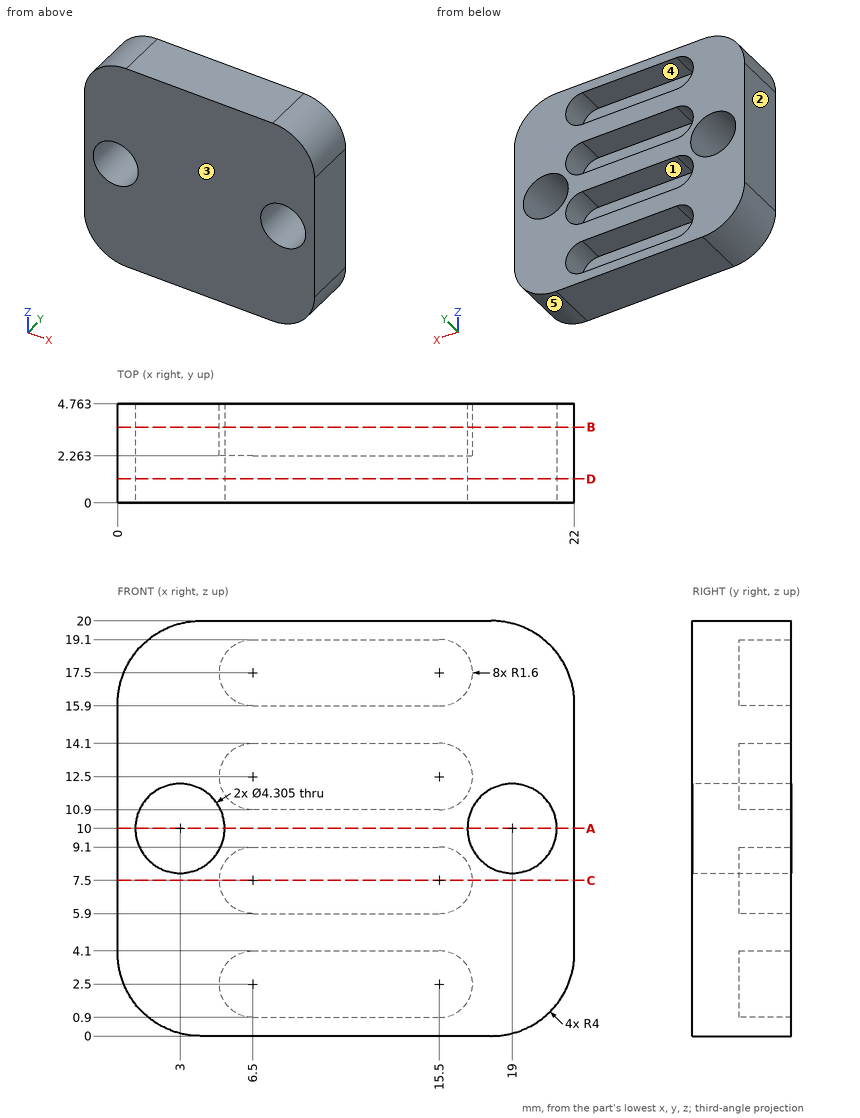
Print and shaded views of the part. All mm, measured from the part's lowest x, y and z. A direction names the side the tool comes from. Give positions to 0.01 mm unless a question says otherwise; leave off trailing zeros. Loops run counter-clockwise (first coordinate to the right, second up) from the corner with the lowest first, then second, coordinate; pieces in that order, holes last. Notation, with made-up numbers: (13.5, 8) -> (40.5, 8) arc R28 ccw to (40.5, 31) -> close; hole circle Ø4 at (-3, -35.75). An arc over 180 degrees is marked (long way). Use a Markdown table: item, result.
1. Which spindle directions (+Z, -Z, +X, -X, +Y, -Y) get a long thin tool onto all of the face, cutting with end or side? Do the marked faces 4 and 5. Say none if no direction does.
Check result:
| item | result |
|---|---|
| face 4 | +Y |
| face 5 | -Z, +X, +Y, -Y |
2. Mould opens along X. For the marked faces 1, 2 and 3 say: pulls with the +X half, pulls with the -X half, needs draft (parallel to the pull), parting line crosses it, or undercut.
Check result:
| item | result |
|---|---|
| face 1 | undercut |
| face 2 | pulls with the -X half |
| face 3 | needs draft |
3. Wall check: L1, parallel to X at y = 1.15, z = 10; L2, parallel to Z at x = 7.25, y = 2.7; L3, parallel to Y at x = 8.5, z = 18.5. Give the ranges that are in metal, low to high. Write a range as [from, to].
Check result:
| item | result |
|---|---|
| L1 | x = [0, 0.85], [5.15, 16.85], [21.15, 22] |
| L2 | z = [0, 0.9], [4.1, 5.9], [9.1, 10.9], [14.1, 15.9], [19.1, 20] |
| L3 | y = [0, 2.26] |
4. Slice it at C-C (z = 7.5). List the corners of the cut face in (x, y).
Check result:
| item | result |
|---|---|
| outline | (0, 0) -> (22, 0) -> (22, 4.76) -> (17.1, 4.76) -> (17.1, 2.26) -> (4.9, 2.26) -> (4.9, 4.76) -> (0, 4.76) -> close |
5. Slice it at A-A (z = 10). List the corners of the cut face in (x, y).
Check result:
| item | result |
|---|---|
| outline | (0, 0) -> (0.85, 0) -> (0.85, 4.76) -> (0, 4.76) -> close; (5.15, 0) -> (16.85, 0) -> (16.85, 4.76) -> (5.15, 4.76) -> close; (21.15, 0) -> (22, 0) -> (22, 4.76) -> (21.15, 4.76) -> close |
6. Slice it at D-D (y = 1.15). List the corners of the cut face in (x, z) (1 decimal).
Check result:
| item | result |
|---|---|
| outline | (0, 4) arc R4 ccw to (4, 0) -> (18, 0) arc R4 ccw to (22, 4) -> (22, 16) arc R4 ccw to (18, 20) -> (4, 20) arc R4 ccw to (0, 16) -> close; hole circle Ø4.3 at (3, 10); hole circle Ø4.3 at (19, 10) |
7. Flat gauge pins, fed straight in: pin 1 (1.5 mm diameter, centred on y = 4.5, z = 18, fed in from +X); pin 2 (1 mm diameter, centred on x = 8.5, z = 7.5, fed in from +Y); pin 3 (4 mm diameter, centred on x = 3, z = 10, fed in from +Y) (3 decimals). Where does each tip first touch, or does it go through?
Check result:
| item | result |
|---|---|
| pin 1 | stops at x = 21.8 |
| pin 2 | stops at y = 2.26 |
| pin 3 | passes through |
8. Slice it at B-B (y = 3.65). List the corners of the cut face in (x, z) (1 decimal).
Check result:
| item | result |
|---|---|
| outline | (0, 4) arc R4 ccw to (4, 0) -> (18, 0) arc R4 ccw to (22, 4) -> (22, 16) arc R4 ccw to (18, 20) -> (4, 20) arc R4 ccw to (0, 16) -> close; hole circle Ø4.3 at (3, 10); hole (6.5, 0.9) -> (15.5, 0.9) arc R1.6 ccw to (15.5, 4.1) -> (6.5, 4.1) arc R1.6 ccw to start; hole (6.5, 5.9) -> (15.5, 5.9) arc R1.6 ccw to (15.5, 9.1) -> (6.5, 9.1) arc R1.6 ccw to start; hole (6.5, 10.9) -> (15.5, 10.9) arc R1.6 ccw to (15.5, 14.1) -> (6.5, 14.1) arc R1.6 ccw to start; hole (6.5, 15.9) -> (15.5, 15.9) arc R1.6 ccw to (15.5, 19.1) -> (6.5, 19.1) arc R1.6 ccw to start; hole circle Ø4.3 at (19, 10) |
